```python
from build123d import *

# Parameters (mm, degrees)
F0_W     = 50.8
F0_H     = 49.806252
F0_R     = 12.7
F1_DEPTH = 25.4
F3_R     = 12.7
F4_DEPTH = 50.8
F6_R     = 12.7
F7_DEPTH = 25.4


with BuildPart() as f1:
    # F0 (on Front) → F1 (new body, symmetric)
    with BuildSketch(Plane.XZ):
        Rectangle(F0_W, F0_H)
        Circle(F0_R, mode=Mode.SUBTRACT)
    extrude(amount=F1_DEPTH, both=True)

    # F3 (on offset) → F4 (cut)
    with BuildSketch(Plane.XY.offset(25.4)):
        Circle(F3_R)
    extrude(amount=-F4_DEPTH, mode=Mode.SUBTRACT)

    # F6 (on offset) → F7 (join)
    with BuildSketch(Plane.YZ.offset(25.4)):
        Circle(F6_R)
    extrude(amount=F7_DEPTH)


solid = f1.part
```
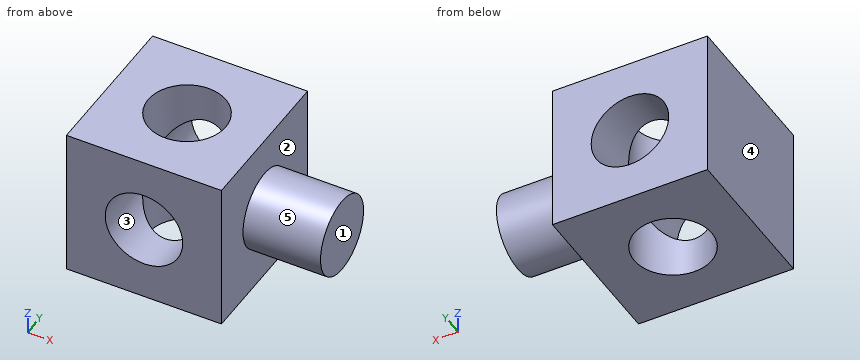
Verification items for the finished model (mm, model axes). Face numbers are marked on the shaded views. A direction names the side the tool comes from. Give positions to 0.01 mm unless a question says otherwise; leave off trailing zeros. Loops run counter-clockwise (first coordinate to the right, second up) from the corner with the lowest first, then second, coordinate; pieces in that order, holes last.
1. Mould release check, pull along X, two halves, no side actions. Record for the marked faces 3, 4 and 5: released by +X, released by -X, zero draft, split by the parting line, or undercut.
2. Thickness scan on line 1 (Z direction, x = 0, y = -17); line 2 (Y direction, x = 0, z = -19). Record the ranges inside material, lowest first.
3. Set-up check for the marked faces 1 and 2: record each of +Z, -Z, +X, -X, +Y, -Y from which the full face is reachable in a straight line by a thin tool's end or side.
4. Section check A-A, the plane x = 0. Enter the section's corners in (y, z), then the cut area to 3 significant figures.
5. Section check D-D, the plane y = 3. Enter the section's corners in (x, z).
6. Section check B-B, the plane y = -22. Enter the section's corners in (x, z).
7. Section check C-C, the plane z = 2.5. Enter the section's corners in (x, y).
8. Go/stop test with flat-tipped pins: pin 1 Ø2 at (x, y) = (32.5, -15) entering from -Z; pin 2 Ø4 at (y, z) = (12, 19.5) entering from +X; pin 3 Ø4 at (x, z) = (36, -6) entering from +Y. Record where each tip stops, or that it passes through.
Geometry says:
1. face 3: undercut
1. face 4: released by -X
1. face 5: zero draft
2. line 1: z = -24.9 to -12.7, 12.7 to 24.9
2. line 2: y = -25.4 to -12.7, 12.7 to 25.4
3. face 1: +Z, -Z, +X, +Y, -Y
3. face 2: +X
4. outline: (-25.4, -24.9) - (-12.7, -24.9) - (-12.7, -12.7) - (-25.4, -12.7) - close; (-25.4, 12.7) - (-12.7, 12.7) - (-12.7, 24.9) - (-25.4, 24.9) - close; (12.7, -24.9) - (25.4, -24.9) - (25.4, -12.7) - (12.7, -12.7) - close; (12.7, 12.7) - (25.4, 12.7) - (25.4, 24.9) - (12.7, 24.9) - close
4. area: 620 mm2
5. outline: (-25.4, -24.9) - (-12.34, -24.9) - (-12.34, -3) arc R12.7 cw to (-12.34, 3) - (-12.34, 24.9) - (-25.4, 24.9) - close; (12.34, -24.9) - (25.4, -24.9) - (25.4, -12.34) - (50.8, -12.34) - (50.8, 12.34) - (25.4, 12.34) - (25.4, 24.9) - (12.34, 24.9) - (12.34, 3) arc R12.7 cw to (12.34, -3) - close
6. outline: (-25.4, -24.9) - (25.4, -24.9) - (25.4, 24.9) - (-25.4, 24.9) - close; hole circle Ø25.4 at (0, 0)
7. outline: (-25.4, -25.4) - (-12.45, -25.4) - (-12.45, -2.5) arc R12.7 cw to (-12.45, 2.5) - (-12.45, 25.4) - (-25.4, 25.4) - close; (12.45, -25.4) - (25.4, -25.4) - (25.4, -12.45) - (50.8, -12.45) - (50.8, 12.45) - (25.4, 12.45) - (25.4, 25.4) - (12.45, 25.4) - (12.45, 2.5) arc R12.7 cw to (12.45, -2.5) - close
8. pin 1: passes through
8. pin 2: stops at x = 25.4
8. pin 3: stops at y = 12.05
